Can you work these out from the model? Positions are in its coordinate system, mm. Face numbers are marked on the shaded views. A direction names the side the tool comes from. Coordinates: 2 decimals unless noted, no trailing zeros. Write each loop counter-clockwise with the first axis right and the second up, starting at its lowest first coordinate (ties: lowest second). Pieces come first, ordered by that corner, then holes. Notation, with made-up numbers: (86.5, 45) - (129.5, 45) arc R26 ccw to (129.5, 69) - close; hole circle Ø6 at (62, 15). An arc over 180 degrees is marked (long way). Use one line per item in the form item = value. Start each with the question number.
(1) If we section it at B-B on x = 11: Please give me the cut outline in (y, z), then the cut area to 3 significant figures.
(2) On a 3-axis mill with a long thin cutter (end or side, diameter ignored), from which of +Z, -Z, +X, -X, +Y, -Y can I reach the whole of each face in a straight line? I mean the marked faces 1 and 2. Say none if no direction works.
(3) Thinking about a two-plate mould opening in X: for the marked faces 3, 4, 5 and 6, which applies, pulls with the +X half, pulls with the -X half, needs draft (parallel to the pull), parting line crosses it, or undercut?
(4) For pin 1 Ø1.1 at (x, z) = (13, -10) entering from +Y; pin 2 Ø0.5 at (x, z) = (26, -4) entering from -Y; pin 3 Ø1.1 at (x, z) = (21.5, -11.5) entering from +Y, each with a flat end and sliding along its axis, tell me the tip position at first contact or that it passes through.
(5) If we section it at A-A on y = 13: Please give me the cut outline in (x, z), then the cut area to 3 significant figures.
(6) If I drill on probe 1 along X at (y, z) = (5.5, -4); probe 2 along X at (y, z) = (1, -9); probe 3 along Z at (x, y) = (26.75, 3.5), over which ranges is the centre line in solid material (lowest first)? Write a range as from..to.
(7) If we section it at C-C on z = -8.25: Please give me the cut outline in (x, y).
```python
from build123d import *

# Parameters (mm, degrees)
EXTRUDE_392_DEPTH      = 16
FILLET_1_R             = 2
SKETCH_6_R             = 0.9
CUT_EXTRUDE_1038_DEPTH = 7
CUT_EXTRUDE_1432_REACH = 43.617
SKETCH_3_W             = 11
SKETCH_3_H             = 3
SKETCH_2_W             = 15.4
SKETCH_2_H             = 1.5
CUT_EXTRUDE_1918_DEPTH = 8
SKETCH_7_W             = 11
SKETCH_7_H             = 2.25
CUT_EXTRUDE_2_DEPTH    = 7.5
SKETCH_8_W             = 14.2
SKETCH_8_H             = 1
CUT_EXTRUDE_3_DEPTH    = 6.5


with BuildPart() as part:
    # Эскиз1 → Extrude 392 (new body)
    with BuildSketch(Plane(origin=(0, 0, 0), x_dir=(1, 0, 0), z_dir=(0, 1, 0))):
        with BuildLine():
            Line((4, 0), (26, 0))
            ThreePointArc((26, 0), (28.828427125, 1.171572875), (30, 4))
            Line((30, 4), (30, 20))
            ThreePointArc((30, 20), (28.828427125, 22.828427125), (26, 24))
            Line((26, 24), (4, 24))
            ThreePointArc((4, 24), (1.171572875, 22.828427125), (0, 20))
            Line((0, 20), (0, 4))
            ThreePointArc((0, 4), (1.171572875, 1.171572875), (4, 0))
        make_face()
    extrude(amount=EXTRUDE_392_DEPTH)

    # Скругление1
    fillet_1_edges = [part.edges().sort_by_distance(p)[0] for p in [
        (1.171572875, 16, -22.828427125),
        (0, 16, -12),
        (1.171572875, 16, -1.171572875),
        (15, 16, 0),
        (28.828427125, 16, -1.171572875),
        (30, 16, -12),
        (28.828427125, 16, -22.828427125),
        (15, 16, -24),
    ]]
    fillet(fillet_1_edges, radius=FILLET_1_R)

    # Эскиз6 → Cut-Extrude 1038 (cut)
    with BuildSketch(Plane.XZ):
        with Locations(Location((4, -4, 0), (0, 0, 270))):
            Circle(SKETCH_6_R)
        with Locations(Location((26, -4, 0), (0, 0, 270))):
            Circle(SKETCH_6_R)
        with Locations(Location((26, -20, 0), (0, 0, 270))):
            Circle(SKETCH_6_R)
        with Locations(Location((4, -20, 0), (0, 0, 270))):
            Circle(SKETCH_6_R)
    extrude(amount=-CUT_EXTRUDE_1038_DEPTH, mode=Mode.SUBTRACT)

    # Эскиз3 → Cut-Extrude 1432 (cut, up to next)
    with BuildSketch(Plane(origin=(0, 16, 0), x_dir=(1, 0, 0), z_dir=(0, 1, 0)), mode=Mode.PRIVATE) as cut_extrude_1432_sk1:
        with Locations((15, 8)):
            Rectangle(SKETCH_3_W, SKETCH_3_H)
    cut_extrude_1432_tool1 = extrude(cut_extrude_1432_sk1.sketch, amount=-CUT_EXTRUDE_1432_REACH, mode=Mode.PRIVATE) & part.part
    add(cut_extrude_1432_tool1.solids().sort_by_distance((15, 16, -8))[0], mode=Mode.SUBTRACT)

    # Эскиз2 → Cut-Extrude 1918 (cut)
    with BuildSketch(Plane(origin=(0, 16, 0), x_dir=(1, 0, 0), z_dir=(0, 1, 0))):
        with Locations((15, 12.5)):
            Rectangle(SKETCH_2_W, SKETCH_2_H)
    extrude(amount=-CUT_EXTRUDE_1918_DEPTH, mode=Mode.SUBTRACT)

    # Эскиз7 → Вырез-Вытянуть2 (cut)
    with BuildSketch(Plane(origin=(0, 16, 0), x_dir=(1, 0, 0), z_dir=(0, 1, 0))):
        with Locations((15, 10.625)):
            Rectangle(SKETCH_7_W, SKETCH_7_H)
    extrude(amount=-CUT_EXTRUDE_2_DEPTH, mode=Mode.SUBTRACT)

    # Эскиз8 → Вырез-Вытянуть3 (cut)
    with BuildSketch(Plane(origin=(0, 16, 0), x_dir=(1, 0, 0), z_dir=(0, 1, 0))):
        with Locations((15, 11.25)):
            Rectangle(SKETCH_8_W, SKETCH_8_H)
    extrude(amount=-CUT_EXTRUDE_3_DEPTH, mode=Mode.SUBTRACT)


solid = part.part
```
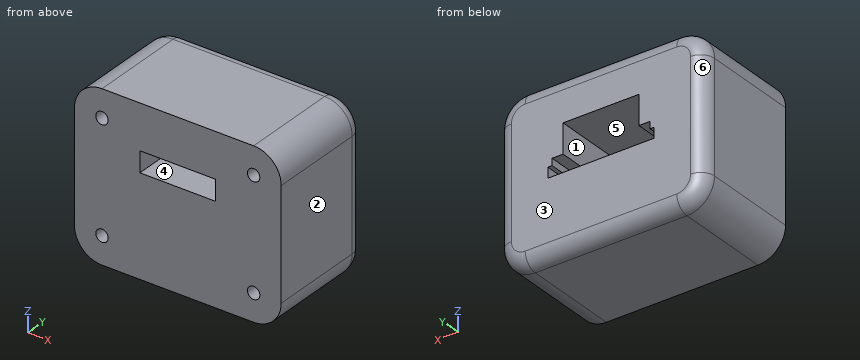
Reported:
q1.outline = (0, -24) - (14, -24) arc R2 ccw to (16, -22) - (16, -13.25) - (8, -13.25) - (8, -11.75) - (8.5, -11.75) - (8.5, -9.5) - (0, -9.5) - close; (0, -6.5) - (16, -6.5) - (16, -2) arc R2 ccw to (14, 0) - (0, 0) - close
q1.area = 305 mm2
q2.face_1 = +Y
q2.face_2 = +Z, -Z, +X, +Y, -Y
q3.face_3 = needs draft
q3.face_4 = undercut
q3.face_5 = undercut
q3.face_6 = pulls with the -X half
q4.pin_1 = 8.5
q4.pin_2 = 7
q4.pin_3 = 9.5
q5.outline = (0, -20) arc R4 ccw to (4, -24) - (26, -24) arc R4 ccw to (30, -20) - (30, -4) arc R4 ccw to (26, 0) - (4, 0) arc R4 ccw to (0, -4) - close; hole (7.3, -13.25) - (22.7, -13.25) - (22.7, -11.75) - (22.1, -11.75) - (22.1, -10.75) - (20.5, -10.75) - (20.5, -6.5) - (9.5, -6.5) - (9.5, -10.75) - (7.9, -10.75) - (7.9, -11.75) - (7.3, -11.75) - close
q5.area = 622 mm2
q6.probe_1 = 0..3.1, 4.9..25.1, 26.9..30
q6.probe_2 = 0..9.5, 20.5..30
q6.probe_3 = -23.93..-20.5, -19.5..-4.5, -3.5..-0.07
q7.outline = (0, 0) - (9.5, 0) - (9.5, 16) - (2, 16) arc R2 ccw to (0, 14) - close; (20.5, 0) - (30, 0) - (30, 14) arc R2 ccw to (28, 16) - (20.5, 16) - close
